from build123d import *

# Parameters (mm, degrees)
SKETCH1_W            = 35
SKETCH1_H            = 70
BOSS_EXTRUDE1_DEPTH  = 3
SKETCH2_W            = 20
SKETCH2_H            = 3
BOSS_EXTRUDE2_DEPTH  = 3
SKETCH3_W            = 20
SKETCH3_H            = 3
BOSS_EXTRUDE3_DEPTH  = 3
SKETCH6_R            = 4.5
CUT_EXTRUDE1_DEPTH   = 10
SKETCH7_R            = 1.5
CUT_EXTRUDE2_DEPTH   = 3
SKETCH8_R            = 1.5
CUT_EXTRUDE3_DEPTH   = 10
SKETCH11_W           = 35
SKETCH11_H           = 60
BOSS_EXTRUDE7_DEPTH  = 3
SKETCH14_W           = 20
SKETCH14_H           = 70
BOSS_EXTRUDE9_DEPTH  = 3
SKETCH15_W           = 3
SKETCH15_H           = 20
BOSS_EXTRUDE10_DEPTH = 3
SKETCH16_W           = 20
SKETCH16_H           = 3
BOSS_EXTRUDE11_DEPTH = 3
SKETCH17_W           = 3
SKETCH17_H           = 20
BOSS_EXTRUDE12_DEPTH = 3


with BuildPart() as part:
    # Sketch1 → Boss-Extrude1 (new body)
    with BuildSketch(Plane(origin=(0, 0, 0), x_dir=(1, 0, 0), z_dir=(0, 1, 0))):
        with Locations((17.5, 35)):
            Rectangle(SKETCH1_W, SKETCH1_H)
    extrude(amount=BOSS_EXTRUDE1_DEPTH)

    # Sketch2 → Boss-Extrude2 (add)
    with BuildSketch(Plane.ZY):
        with Locations((-60, 1.5)):
            Rectangle(SKETCH2_W, SKETCH2_H)
    extrude(amount=BOSS_EXTRUDE2_DEPTH)

    # Sketch3 → Boss-Extrude3 (add)
    with BuildSketch(Plane.ZY):
        with Locations((-20, 1.5)):
            Rectangle(SKETCH3_W, SKETCH3_H)
    extrude(amount=BOSS_EXTRUDE3_DEPTH)

    # Sketch6 → Cut-Extrude1 (cut)
    with BuildSketch(Plane(origin=(0, 3, 0), x_dir=(1, 0, 0), z_dir=(0, 1, 0))):
        with Locations((17.5, 35)):
            Circle(SKETCH6_R)
    extrude(amount=-CUT_EXTRUDE1_DEPTH, mode=Mode.SUBTRACT)

    # Sketch7 → Cut-Extrude2 (cut)
    with BuildSketch(Plane.XZ):
        with Locations((17.5, -25)):
            Circle(SKETCH7_R)
    extrude(amount=-CUT_EXTRUDE2_DEPTH, mode=Mode.SUBTRACT)

    # Sketch8 → Cut-Extrude3 (cut)
    with BuildSketch(Plane.XZ):
        with Locations((17.5, -45)):
            Circle(SKETCH8_R)
    extrude(amount=-CUT_EXTRUDE3_DEPTH, mode=Mode.SUBTRACT)

    # Sketch11 → Boss-Extrude7 (add)
    with BuildSketch(Plane(origin=(0, 3, 0), x_dir=(1, 0, 0), z_dir=(0, 1, 0))):
        with Locations((17.5, -30)):
            Rectangle(SKETCH11_W, SKETCH11_H)
    extrude(amount=-BOSS_EXTRUDE7_DEPTH)

    # Sketch14 → Boss-Extrude9 (add)
    with BuildSketch(Plane(origin=(0, 3, 0), x_dir=(1, 0, 0), z_dir=(0, 1, 0))):
        with Locations((45, 35)):
            Rectangle(SKETCH14_W, SKETCH14_H)
    extrude(amount=-BOSS_EXTRUDE9_DEPTH)

    # Sketch15 → Boss-Extrude10 (add)
    with BuildSketch(Plane(origin=(0, 3, 0), x_dir=(1, 0, 0), z_dir=(0, 1, 0))):
        with Locations((56.5, 60)):
            Rectangle(SKETCH15_W, SKETCH15_H)
        with Locations((56.5, 20)):
            Rectangle(SKETCH15_W, SKETCH15_H)
    extrude(amount=-BOSS_EXTRUDE10_DEPTH)

    # Sketch16 → Boss-Extrude11 (add)
    with BuildSketch(Plane(origin=(0, 3, 0), x_dir=(1, 0, 0), z_dir=(0, 1, 0))):
        with Locations((30, 71.5)):
            Rectangle(SKETCH16_W, SKETCH16_H)
    extrude(amount=-BOSS_EXTRUDE11_DEPTH)

    # Sketch17 → Boss-Extrude12 (add)
    with BuildSketch(Plane(origin=(0, 3, 0), x_dir=(1, 0, 0), z_dir=(0, 1, 0))):
        with Locations((36.5, -40)):
            Rectangle(SKETCH17_W, SKETCH17_H)
        with Locations((-1.5, -20)):
            Rectangle(SKETCH17_W, SKETCH17_H)
    extrude(amount=-BOSS_EXTRUDE12_DEPTH)


solid = part.part
The listing builds one solid part. Answer for the finished solid, in the listing's coordinates (mm). A direction names the side the tool comes from. Coordinates: 2 decimals unless noted, no trailing zeros. Write each loop counter-clockwise with the first axis right and the second up, starting at its lowest first coordinate (ties: lowest second). Pieces come first, ordered by that corner, then holes. Notation, with made-up numbers: (34.25, -3.5) - (88.25, -3.5) arc R24 ccw to (88.25, 19.5) - close; hole circle Ø10 at (25.5, 12.5). An arc over 180 degrees is marked (long way). Put each result on its own line as item: value.
1. Flat-ended cylindrical pins translate along their axes: pin 1 Ø1.5 at (x, y) = (56, 1) entering from -Z; pin 2 Ø1.5 at (y, z) = (1.5, -4.5) entering from +X; pin 3 Ø0.9 at (x, y) = (44.5, 1) entering from +Z. Find the tip coordinate at first contact, or state that the pin passes through.
Answer sheet:
pin 1: stops at z = -70
pin 2: stops at x = 55
pin 3: stops at z = 0
2. Determine the mould class of faces 6 (the face through (16.52, 1.52, -30.61)), 7 (the face through (-1, 1, -30)), 8 (the face through (35, 2, 55)), 9 (the face through (56, 2, -10)) for opening direction Z: pulls with the +Z half, pulls with the -Z half, needs draft (parallel to the pull), parting line crosses it, or undercut.
Answer sheet:
face 6: undercut
face 7: undercut
face 8: needs draft
face 9: pulls with the +Z half
3. The part is cut by section B-B on x = 17.5. Give the vertices of the cut face in (y, z).
Answer sheet:
outline: (0, -70) - (3, -70) - (3, -46.5) - (0, -46.5) - close; (0, -43.5) - (3, -43.5) - (3, -39.5) - (0, -39.5) - close; (0, -30.5) - (3, -30.5) - (3, -26.5) - (0, -26.5) - close; (0, -23.5) - (3, -23.5) - (3, 60) - (0, 60) - close
4. The part is cut by section D-D on z = 46. Give the vertices of the cut face in (x, y).
Answer sheet:
outline: (0, 0) - (38, 0) - (38, 3) - (0, 3) - close
5. A tool of negligible diameter and unlimited length cuts with its end or side. For faces 1 (the face through (8, 2, -70)), 2 (the face through (0, 2, 45)), 3 (the face through (0, 2, 0)), 4 (the face through (40, 2, -71)), 5 (the face through (36, 2, 50)), from which of +Z, -Z, +X, -X, +Y, -Y can it reach the whole face along a straight path? Write none if from no direction.
Answer sheet:
face 1: -Z, -X, +Y, -Y
face 2: +Z, -X, +Y, -Y
face 3: -X, +Y, -Y
face 4: -Z, +X, +Y, -Y
face 5: +Z, +X, +Y, -Y
6. Find the intervals of material crossed by line 1 along Z through (x, y) = (17.5, 1); line 2 along X through (y, z) = (2.25, -35); line 3 along Z through (x, y) = (17, 0.3), in increasing order. Write a range as from..to.
Answer sheet:
line 1: z = -70..-46.5, -43.5..-39.5, -30.5..-26.5, -23.5..60
line 2: x = 0..13, 22..55
line 3: z = -70..-46.41, -43.59..-39.47, -30.53..-26.41, -23.59..60
7. The part is cut by section A-A on z = -35. Give the vertices of the cut face in (x, y), plus the area to 3 significant figures.
Answer sheet:
outline: (0, 0) - (13, 0) - (13, 3) - (0, 3) - close; (22, 0) - (55, 0) - (55, 3) - (22, 3) - close
area: 138 mm^2
8. The part is cut by section C-C on y = 2.55. State how many separate pieces and enclosed holes the cut face has, plus the area to 3 significant figures.
Answer sheet:
separate pieces: 1
enclosed holes: 3
area: 6,290 mm^2
